Autodesk Fusion 360 part; units mm, degrees
sketch "Sketch1" plane through (0, 0, 0) normal (0, 0, 1) x (1, 0, 0)
  line L0 (18, 0) -> (18, 40)
  line L1 (18, 40) -> (-18, 40)
  line L2 (-18, 40) -> (-18, 0)
  arc A0 (18, 40) -> (-18, 40) centre (0, 40) ccw
  line L3 (-10.15, 8) -> (10.15, 8)
  line L4 (10.15, 8) -> (10.15, 49)
  line L5 (-10.15, 49) -> (-10.15, 8)
  line L6 (3.75, 49) -> (3.75, 55)
  line L7 (3.75, 55) -> (-3.75, 55)
  line L8 (-3.75, 55) -> (-3.75, 49)
  line L9 (10.15, 49) -> (3.75, 49)
  line L10 (-3.75, 49) -> (-10.15, 49)
  circle A1 centre (5.15, 52.75) radius 1
  line L11 (0, 55) -> (0, 40)
  line L12 (10.15, 28.5) -> (-10.15, 28.5)
  circle A2 centre (-5.15, 52.75) radius 1
  circle A3 centre (-5.15, 4.25) radius 1
  circle A4 centre (5.15, 4.25) radius 1
  line L13 (-18, 0) -> (18, 0)
  circle A5 centre (-5.15, -52.75) radius 1
  circle A6 centre (5.15, -4.25) radius 1
  line L14 (-10.15, -8) -> (10.15, -8)
  line L15 (18, 0) -> (18, -40)
  circle A7 centre (5.15, -52.75) radius 1
  line L16 (-10.15, -49) -> (-10.15, -8)
  circle A8 centre (-5.15, -4.25) radius 1
  line L17 (0, -55) -> (0, -40)
  line L18 (3.75, -49) -> (3.75, -55)
  line L19 (18, -40) -> (-18, -40)
  line L20 (-3.75, -55) -> (-3.75, -49)
  line L21 (10.15, -28.5) -> (-10.15, -28.5)
  line L22 (10.15, -8) -> (10.15, -49)
  line L23 (3.75, -55) -> (-3.75, -55)
  line L24 (10.15, -49) -> (3.75, -49)
  line L25 (-18, -40) -> (-18, 0)
  line L26 (-3.75, -49) -> (-10.15, -49)
  arc A9 (-18, -40) -> (18, -40) centre (0, -40) ccw
  point P0 (0, 40)
  point P1 (0, 8)
  point P2 (0, 55)
  point P3 (0, -55)
  point P4 (0, -8)
  point P5 (0, -40)
  dimension "d1" = 40
  dimension "d2" = 36
  dimension "d3" = 41
  dimension "d4" = 20.3
  dimension "d5" = 7.5
  dimension "d6" = 6
  dimension "d7" = 2
  dimension "d8" = 5
  dimension "d9" = 3.75
  dimension "d10" = 15
extrude "Extrude1" add sketch "Sketch1" along normal blind 8 contours L0 L1 L2 L3 L4 L5 L13 | L13 L14 L15 L16 L19 L22 L25 | L1 A0 L4 L5 L6 L7 L8 L9 L10 | L16 L18 L19 L20 L22 L23 L24 L26 A9
sketch "Sketch2" plane through (0, 0, 8) normal (0, 0, 1) x (-1, 0, 0)
  circle A0 centre (-5.15, -4.25) radius 1
  circle A1 centre (-5.15, -52.75) radius 1
  circle A2 centre (5.15, -52.75) radius 1
  line L0 (10.15, -49) -> (3.75, -49)
  line L1 (3.75, -49) -> (3.75, -55)
  line L2 (3.75, -55) -> (-3.75, -55)
  line L3 (-3.75, -55) -> (-3.75, -49)
  line L4 (-3.75, -49) -> (-10.15, -49)
  line L5 (-10.15, -49) -> (-10.15, -8)
  line L6 (-10.15, -8) -> (10.15, -8)
  line L7 (10.15, -8) -> (10.15, -49)
  circle A3 centre (5.15, -4.25) radius 1
  line L8 (-18, 40) -> (-18, -40)
  arc A4 (-18, -40) -> (18, -40) centre (0, -40) ccw
  line L9 (18, -40) -> (18, 40)
  circle A5 centre (14.075, -39) radius 1.6
  circle A6 centre (14.075, -39) radius 2.6
  line L10 (18, -39) -> (10.15, -39)
  line L11 (0, -55) -> (0, -8)
  line L12 (10.15, -28.5) -> (-10.15, -28.5)
  circle A7 centre (14.075, -18) radius 2.6
  circle A8 centre (14.075, -18) radius 1.6
  circle A9 centre (-14.075, -39) radius 1.6
  circle A10 centre (-14.075, -39) radius 2.6
  circle A11 centre (-14.075, -18) radius 1.6
  circle A12 centre (-14.075, -18) radius 2.6
  circle A13 centre (-5.15, 52.75) radius 1
  line L13 (3.75, 55) -> (3.75, 49)
  line L14 (3.75, 49) -> (10.15, 49)
  line L15 (10.15, 49) -> (10.15, 8)
  line L16 (10.15, 8) -> (-10.15, 8)
  line L17 (-10.15, 8) -> (-10.15, 49)
  line L18 (-10.15, 49) -> (-3.75, 49)
  line L19 (-3.75, 49) -> (-3.75, 55)
  line L20 (-3.75, 55) -> (3.75, 55)
  circle A14 centre (5.15, 52.75) radius 1
  circle A15 centre (5.15, 4.25) radius 1
  circle A16 centre (-5.15, 4.25) radius 1
  arc A17 (18, 40) -> (-18, 40) centre (0, 40) ccw
  line L21 (18, 0) -> (-18, 0)
  circle A18 centre (14.075, 18) radius 2.6
  circle A19 centre (14.075, 18) radius 1.6
  circle A20 centre (14.075, 39) radius 1.6
  circle A21 centre (14.075, 39) radius 2.6
  circle A22 centre (-14.075, 39) radius 1.6
  circle A23 centre (-14.075, 39) radius 2.6
  circle A24 centre (-14.075, 18) radius 1.6
  circle A25 centre (-14.075, 18) radius 2.6
  point P0 (14.075, -39)
  dimension "d25" = 3.2
  dimension "d26" = 5.2
  dimension "d28" = 10
extrude "Extrude2" cut sketch "Sketch2" against normal up to surface (8 mm away) contours A5 L10 | A5 L10 | A8 | A9 | A11 | A19 | A20 | A22 | A24
extrude "Extrude3" cut sketch "Sketch2" against normal blind 4 contours A5 A6 L10 | A5 A6 L10 | A10 | A21 | A23
sketch "Sketch3" plane through (0, 0, 0) normal (0, 0, 1) x (-1, 0, 0)
  circle A0 centre (-14.075, -18) radius 1.6
  circle A1 centre (14.075, 18) radius 1.6
  circle A2 centre (14.075, -18) radius 1.6
  circle A3 centre (-14.075, 18) radius 1.6
  circle A4 centre (-14.075, -39) radius 1.6
  circle A5 centre (14.075, 39) radius 1.6
  circle A6 centre (14.075, -39) radius 1.6
  circle A7 centre (-14.075, 39) radius 1.6
  circle A8 centre (-5.15, -4.25) radius 1
  circle A9 centre (-5.15, -52.75) radius 1
  circle A10 centre (-5.15, 52.75) radius 1
  circle A11 centre (5.15, -4.25) radius 1
  line L0 (3.75, 49) -> (3.75, 55)
  line L1 (3.75, 55) -> (-3.75, 55)
  line L2 (-3.75, 55) -> (-3.75, 49)
  line L3 (-3.75, 49) -> (-10.15, 49)
  line L4 (-10.15, 49) -> (-10.15, 8)
  line L5 (-10.15, 8) -> (10.15, 8)
  line L6 (10.15, 8) -> (10.15, 49)
  line L7 (10.15, 49) -> (3.75, 49)
  circle A12 centre (5.15, -52.75) radius 1
  circle A13 centre (5.15, 52.75) radius 1
  circle A14 centre (5.15, 4.25) radius 1
  circle A15 centre (-5.15, 4.25) radius 1
  line L8 (3.75, -49) -> (10.15, -49)
  line L9 (10.15, -49) -> (10.15, -8)
  line L10 (10.15, -8) -> (-10.15, -8)
  line L11 (-10.15, -8) -> (-10.15, -49)
  line L12 (-10.15, -49) -> (-3.75, -49)
  line L13 (-3.75, -49) -> (-3.75, -55)
  line L14 (-3.75, -55) -> (3.75, -55)
  line L15 (3.75, -55) -> (3.75, -49)
  line L16 (-18, -40) -> (-18, 40)
  arc A16 (18, 40) -> (-18, 40) centre (0, 40) ccw
  line L17 (18, 40) -> (18, -40)
  arc A17 (-18, -40) -> (18, -40) centre (0, -40) ccw
  circle A18 centre (-14.075, -18) radius 2.6
  circle A19 centre (-14.075, 18) radius 2.6
  circle A20 centre (14.075, 18) radius 2.6
  circle A21 centre (14.075, -18) radius 2.6
extrude "Extrude4" cut sketch "Sketch3" along normal blind 4 contours A18 | A19 | A20 | A21
Geometry check sheet. Reference: the model listing, model coordinates, mm. A direction names the side the tool comes from. Coordinates: 2 decimals unless noted, no trailing zeros. Order: outer loops, then holes, each group sorted by start corner. A loop starts at its lowest first (then second) coordinate and runs counter-clockwise, first axis right, second up. Notation, with made-up numbers: (39.25, 38.5) - (77.25, 38.5) arc R26 cw to (77.25, 62.5) - close; hole circle Ø7 at (24.5, 75.25). An arc over 180 degrees is marked (long way). Answer in a Markdown table with one row per item. Add a question column.
1. Draft check along X on faces 4 (the face through (3.75, -52, 4)), 5 (the face through (-18, 1, 4)). Enter one of: +X half, -X half, draft (parallel to the pull), parting line (faces both ways), or undercut.
2. Section check A-A (x = 0). Enter the section's corners in (y, z).
3. Gauge pin test, flat ends, axial feed: pin 1 Ø2.5 at (x, y) = (-14.5, -17.5) entering from -Z; pin 2 Ø3 at (y, z) = (-53, 3) entering from -X; pin 3 Ø1.6 at (x, y) = (-15, 38.5) entering from +Z; pin 4 Ø3 at (x, y) = (14.075, 39) entering from -Z. Record the tip position at first contact, or that the pin passes through.
4. Material ranges on L1, parallel to X at y = -18, z = 2.85 (3 decimals); L2, parallel to X at y = 18, z = 5.5 (3 decimals); L3, parallel to X at y = 15, z = 7, recorded low to high. Write a range as [from, to].
5. Section check B-B (y = 4.25). Enter the section's corners in (x, z).
6. Section check C-C (y = -18). Enter the section's corners in (x, z) (3 decimals), plus the area to 3 significant figures.
7. Access from +Z, -Z, +X, -X, +Y, -Y to the whole of each face (thin tool, end or side, straight path). Record for faces 1 (the face through (16.672, -17.886, 1.972)), 2 (the face through (14.639, -36.462, 6.028)), 3 (the face through (7, -49, 4)).
8. Section check D-D (x = -5.15). Enter the section's corners in (y, z).
Data:
| question | item | result |
|---|---|---|
| 1 | face 4 | undercut |
| 1 | face 5 | -X half |
| 2 | outline | (-58, 0) - (-55, 0) - (-55, 8) - (-58, 8) - close; (-8, 0) - (8, 0) - (8, 8) - (-8, 8) - close; (55, 0) - (58, 0) - (58, 8) - (55, 8) - close |
| 3 | pin 1 | stops at z = 4 |
| 3 | pin 2 | stops at x = -13.85 |
| 3 | pin 3 | stops at z = 4 |
| 3 | pin 4 | passes through |
| 4 | L1 | x = [-18, -16.675], [-11.475, -10.15], [10.15, 11.475], [16.675, 18] |
| 4 | L2 | x = [-18, -15.675], [-12.475, -10.15], [10.15, 12.475], [15.675, 18] |
| 4 | L3 | x = [-18, -10.15], [10.15, 18] |
| 5 | outline | (-18, 0) - (-6.15, 0) - (-6.15, 8) - (-18, 8) - close; (-4.15, 0) - (4.15, 0) - (4.15, 8) - (-4.15, 8) - close; (6.15, 0) - (18, 0) - (18, 8) - (6.15, 8) - close |
| 6 | outline | (-18, 0) - (-16.675, 0) - (-16.675, 4) - (-15.675, 4) - (-15.675, 8) - (-18, 8) - close; (-12.475, 4) - (-11.475, 4) - (-11.475, 0) - (-10.15, 0) - (-10.15, 8) - (-12.475, 8) - close; (10.15, 0) - (11.475, 0) - (11.475, 4) - (12.475, 4) - (12.475, 8) - (10.15, 8) - close; (15.675, 4) - (16.675, 4) - (16.675, 0) - (18, 0) - (18, 8) - (15.675, 8) - close |
| 6 | area | 58.4 mm² |
| 7 | face 1 | -Z |
| 7 | face 2 | +Z |
| 7 | face 3 | +Z, -Z |
| 8 | outline | (-57.25, 0) - (-53.75, 0) - (-53.75, 8) - (-57.25, 8) - close; (-51.75, 0) - (-49, 0) - (-49, 8) - (-51.75, 8) - close; (-8, 0) - (-5.25, 0) - (-5.25, 8) - (-8, 8) - close; (-3.25, 0) - (3.25, 0) - (3.25, 8) - (-3.25, 8) - close; (5.25, 0) - (8, 0) - (8, 8) - (5.25, 8) - close; (49, 0) - (51.75, 0) - (51.75, 8) - (49, 8) - close; (53.75, 0) - (57.25, 0) - (57.25, 8) - (53.75, 8) - close |
